Autodesk Inventor part; units mm, degrees
ref_plane "РабПлоскость1" through (0, 20, 0) normal (0, -1, 0) x (1, 0, 0)
ref_plane "РабПлоскость2" through (0, 25, 0) normal (0, -1, 0) x (1, 0, 0)
ref_plane "YZ Plane" through (0, 0, 0) normal (1, 0, 0) x (0, 1, 0)
sketch "Эскиз1" plane through (0, 0, 0) normal (0, 1, 0) x (-1, 0, 0)
  circle A0 centre (0, 0) radius 15
  dimension "d0" = 30
extrude "Выдавливание1" add sketch "Эскиз1" along normal blind 55
ref_plane "РабПлоскость1" through (0, 20, 0) normal (0, -1, 0) x (1, 0, 0)
sketch "Эскиз5" plane through (0, 20, 0) normal (0, -1, 0) x (1, 0, 0)
  point P0 (0, 0)
  point P1 (0, 0)
hole "Отверстие2" at (0, 20, 0) direction (0, 1, 0) diameter 20 depth 5
ref_plane "РабПлоскость2" through (0, 25, 0) normal (0, -1, 0) x (1, 0, 0)
sketch "Эскиз6" plane through (0, 25, 0) normal (0, -1, 0) x (1, 0, 0)
  point P0 (0, 0)
  point P1 (0, 0)
hole "Отверстие3" at (0, 25, 0) direction (0, 1, 0) diameter 12 end through all countersink diameter 20 countersink angle 90
sketch "Эскиз7" plane through (0, 0, 0) normal (0, -1, 0) x (1, 0, 0)
  circle A0 centre (0, 0) radius 10
  dimension "d24" = 20
extrude "Выдавливание2" cut sketch "Эскиз7" against normal blind 20
thread "Резьба1"
Geometry: final body of the model. Coordinates: model frame, mm. Coordinates: 2 decimals unless noted, no trailing zeros. Order: outer loops, then holes, each group sorted by start corner. A loop starts at its lowest first (then second) coordinate and runs counter-clockwise, first axis right, second up.
1) First-contact query: P1, Ø2, axis at x = 0, z = -3.5, coming from the +Y side; P2, Ø12, axis at x = -4, z = 3.5, coming from the +Y side; P3, Ø8, axis at x = 6, y = 6, coming from the +Z side; P4, Ø1, axis at x = 2.5, y = 10.5, coming from the -Z side. Flat tips, straight axial feed; report the tip coordinate or a pass-through.
Result sheet:
P1: passes through
P2: stops at y = 55
P3: stops at z = 14.87
P4: stops at z = -14.87
2) Section A-A (z = 0). Return loops of the section in (x, y), then the cut area to 3 significant figures.
Result sheet:
outline: (-15, 0) - (-10, 0) - (-10, 25) - (-6, 29) - (-6, 55) - (-15, 55) - close; (6, 29) - (10, 25) - (10, 0) - (15, 0) - (15, 55) - (6, 55) - close
area: 774 mm2
3) Section C-C (y = 14). Return loops of the section in (x, z), then the cut area to 3 significant figures.
Result sheet:
outline: circle Ø30 at (0, 0); hole circle Ø20 at (0, 0)
area: 393 mm2
4) Draft query along X for faces 1 (the cylindrical face through (14.985, 27.115, -0.66)), 2 (the flat face through (-3, 0, -10)), 3 (the conical face through (-5.55, 28.75, -2.88)). Return one class per face: released by +X, released by -X, zero draft, split by the parting line, or undercut.
Result sheet:
face 1: split by the parting line
face 2: zero draft
face 3: undercut
5) Ray query, probe 1 along Z at (x, y) = (0, 6.25); probe 2 along X at (y, z) = (3, -5.5); probe 3 along X at (y, z) = (51, -0.5). Return the intervals inside material, ascending.
Result sheet:
probe 1: z = -15 to -10, 10 to 15
probe 2: x = -13.96 to -8.35, 8.35 to 13.96
probe 3: x = -14.99 to -5.98, 5.98 to 14.99
6) Section B-B (x = 0). Return loops of the section in (y, z).
Result sheet:
outline: (0, -15) - (55, -15) - (55, -6) - (29, -6) - (25, -10) - (0, -10) - close; (0, 10) - (25, 10) - (29, 6) - (55, 6) - (55, 15) - (0, 15) - close
7) Section D-D (x = 12). Return loops of the section in (y, z), then the cut area to 3 significant figures.
Result sheet:
outline: (0, -9) - (55, -9) - (55, 9) - (0, 9) - close
area: 990 mm2
